```python
from build123d import *

# Parameters (mm, degrees)
SKETCH1_W             = 23.495
SKETCH1_H             = 30.48
BOSS_EXTRUDE1_DEPTH   = 3.3274
SKETCH2_W             = 21.971
SKETCH2_H             = 28.956
BOSS_EXTRUDE2_DEPTH   = 17.78
SKETCH3_W             = 16.2306
SKETCH3_H             = 24.3332
CUT_EXTRUDE1_DEPTH    = 16.51
CHAMFER1_SIZE         = 4.445
SKETCH4_W             = 4.064
SKETCH4_H             = 2.032
BOSS_EXTRUDE3_DEPTH   = 16.002
CHAMFER2_SIZE         = 1.27
CHAMFER2_SIZE2        = 0.508
CHAMFER2_PART_2_SIZE  = 1.27
CHAMFER2_PART_2_SIZE2 = 0.508
CHAMFER3_SIZE         = 1.27
CHAMFER3_SIZE2        = 0.508
CHAMFER3_PART_2_SIZE  = 1.27
CHAMFER3_PART_2_SIZE2 = 0.508
SKETCH5_W             = 4.064
SKETCH5_H             = 2.032
BOSS_EXTRUDE4_DEPTH   = 12.446
CHAMFER4_SIZE         = 1.27
CHAMFER4_SIZE2        = 0.508
CHAMFER4_PART_2_SIZE  = 1.27
CHAMFER4_PART_2_SIZE2 = 0.508
CHAMFER4_PART_3_SIZE  = 1.27
CHAMFER4_PART_3_SIZE2 = 0.508
CHAMFER4_PART_4_SIZE  = 1.27
CHAMFER4_PART_4_SIZE2 = 0.508
CHAMFER5_SIZE         = 0.508
CHAMFER5_SIZE2        = 1.27


with BuildPart() as part:
    # Sketch1 → Boss-Extrude1 (new body)
    with BuildSketch(Plane(origin=(0, 0, 0), x_dir=(0, 0, -1), z_dir=(1, 0, 0))):
        Rectangle(SKETCH1_W, SKETCH1_H)
    extrude(amount=BOSS_EXTRUDE1_DEPTH)

    # Sketch2 → Boss-Extrude2 (add)
    with BuildSketch(Plane.ZY):
        Rectangle(SKETCH2_W, SKETCH2_H)
    extrude(amount=BOSS_EXTRUDE2_DEPTH)

    # Sketch3 → Cut-Extrude1 (cut)
    with BuildSketch(Plane(origin=(3.3274, 0, 0), x_dir=(0, 0, -1), z_dir=(1, 0, 0))):
        Rectangle(SKETCH3_W, SKETCH3_H)
    extrude(amount=-CUT_EXTRUDE1_DEPTH, mode=Mode.SUBTRACT)

    # Chamfer1
    chamfer1_edges = [part.edges().sort_by_distance(p)[0] for p in [
        (-4.9276, -12.1666, 8.1153),
        (-4.9276, 12.1666, 8.1153),
    ]]
    chamfer(chamfer1_edges, length=CHAMFER1_SIZE)

    # Sketch4 → Boss-Extrude3 (add)
    with BuildSketch(Plane(origin=(2.8194, 0, 0), x_dir=(0, 0, -1), z_dir=(1, 0, 0))):
        with Locations((-4.155513801, 0.215773581)):
            Rectangle(SKETCH4_W, SKETCH4_H)
    extrude(amount=-BOSS_EXTRUDE3_DEPTH)

    # Chamfer2
    chamfer2_edges = [part.edges().sort_by_distance(p)[0] for p in [
        (2.8194, 1.231773581, 4.155513801),
    ]]
    chamfer2_side = [part.faces().sort_by_distance(p)[0] for p in [
        (-5.1816, 1.231773581, 4.155513801),
    ]]
    chamfer(chamfer2_edges, length=CHAMFER2_SIZE, length2=CHAMFER2_SIZE2, reference=chamfer2_side[0])

    # Chamfer2 part 2
    chamfer2_part_2_edges = [part.edges().sort_by_distance(p)[0] for p in [
        (2.8194, -0.800226419, 4.155513801),
    ]]
    chamfer2_part_2_side = [part.faces().sort_by_distance(p)[0] for p in [
        (-5.1816, -0.800226419, 4.155513801),
    ]]
    chamfer(chamfer2_part_2_edges, length=CHAMFER2_PART_2_SIZE, length2=CHAMFER2_PART_2_SIZE2, reference=chamfer2_part_2_side[0])

    # Chamfer3
    chamfer3_edges = [part.edges().sort_by_distance(p)[0] for p in [
        (2.8194, 0.215773581, 2.123513801),
    ]]
    chamfer3_side = [part.faces().sort_by_distance(p)[0] for p in [
        (-5.334994062, 0.215773581, 2.123513801),
    ]]
    chamfer(chamfer3_edges, length=CHAMFER3_SIZE, length2=CHAMFER3_SIZE2, reference=chamfer3_side[0])

    # Chamfer3 part 2
    chamfer3_part_2_edges = [part.edges().sort_by_distance(p)[0] for p in [
        (2.8194, 0.215773581, 6.187513801),
    ]]
    chamfer3_part_2_side = [part.faces().sort_by_distance(p)[0] for p in [
        (-5.334994062, 0.215773581, 6.187513801),
    ]]
    chamfer(chamfer3_part_2_edges, length=CHAMFER3_PART_2_SIZE, length2=CHAMFER3_PART_2_SIZE2, reference=chamfer3_part_2_side[0])

    # Sketch5 → Boss-Extrude4 (add)
    with BuildSketch(Plane(origin=(-0.7366, 0, 0), x_dir=(0, 0, -1), z_dir=(1, 0, 0))):
        with Locations((1.9685, 7.0358)):
            Rectangle(SKETCH5_W, SKETCH5_H)
    boss_extrude4 = extrude(amount=-BOSS_EXTRUDE4_DEPTH)

    # Chamfer4
    chamfer4_edges = [part.edges().sort_by_distance(p)[0] for p in [
        (-0.7366, 7.0358, -4.0005),
    ]]
    chamfer4_side = [part.faces().sort_by_distance(p)[0] for p in [
        (-6.9596, 7.0358, -4.0005),
    ]]
    chamfer(chamfer4_edges, length=CHAMFER4_SIZE, length2=CHAMFER4_SIZE2, reference=chamfer4_side[0])

    # Chamfer4 part 2
    chamfer4_part_2_edges = [part.edges().sort_by_distance(p)[0] for p in [
        (-0.7366, 8.0518, -1.9685),
    ]]
    chamfer4_part_2_side = [part.faces().sort_by_distance(p)[0] for p in [
        (-6.9596, 8.0518, -1.9685),
    ]]
    chamfer(chamfer4_part_2_edges, length=CHAMFER4_PART_2_SIZE, length2=CHAMFER4_PART_2_SIZE2, reference=chamfer4_part_2_side[0])

    # Chamfer4 part 3
    chamfer4_part_3_edges = [part.edges().sort_by_distance(p)[0] for p in [
        (-0.7366, 7.0358, 0.0635),
    ]]
    chamfer4_part_3_side = [part.faces().sort_by_distance(p)[0] for p in [
        (-6.9596, 7.0358, 0.0635),
    ]]
    chamfer(chamfer4_part_3_edges, length=CHAMFER4_PART_3_SIZE, length2=CHAMFER4_PART_3_SIZE2, reference=chamfer4_part_3_side[0])

    # Chamfer4 part 4
    chamfer4_part_4_edges = [part.edges().sort_by_distance(p)[0] for p in [
        (-0.7366, 6.0198, -1.9685),
    ]]
    chamfer4_part_4_side = [part.faces().sort_by_distance(p)[0] for p in [
        (-6.9596, 6.0198, -1.9685),
    ]]
    chamfer(chamfer4_part_4_edges, length=CHAMFER4_PART_4_SIZE, length2=CHAMFER4_PART_4_SIZE2, reference=chamfer4_part_4_side[0])

    # Mirror7: Boss-Extrude4 across plane
    add(boss_extrude4.mirror(Plane.ZX))

    # Chamfer5
    chamfer5_edges = [part.edges().sort_by_distance(p)[0] for p in [
        (-0.7366, -7.0358, -4.0005),
        (-0.7366, -8.0518, -1.9685),
        (-0.7366, -7.0358, 0.0635),
        (-0.7366, -6.0198, -1.9685),
    ]]
    chamfer5_side = [part.faces().sort_by_distance(p)[0] for p in [
        (-0.7366, -7.0358, -1.9685),
    ]]
    chamfer(chamfer5_edges, length=CHAMFER5_SIZE, length2=CHAMFER5_SIZE2, reference=chamfer5_side[0])


solid = part.part
```
For this review, take the finished solid that the model builds, in its own axes (mm). A direction names the side the tool comes from. Round coordinates to 2 decimals unless told otherwise and drop trailing zeros. Write each loop counter-clockwise with the first axis right and the second up, starting at its lowest first coordinate (ties: lowest second). Pieces come first, ordered by that corner, then holes. Notation, with made-up numbers: M 9.5,-33.5 L 25.5,-33.5 A27 cw 25.5,-6.5 Z; hole C 49,76.5 d9. An arc over 180 degrees is marked long. One line per item, written item: value. Start each with the question number.
(1) Wall thickness on line 1 (Y direction, x = -9, z = 0); line 2 (Y direction, x = -2.25, z = 3.25); line 3 (Z direction, x = -1.75, y = 3): over which ranges is each line inside the solid? List them lowest first.
(2) We need section B-B (y = 13). Give the boundary of the cut face in (x, z).
(3) The part is to be moulded in two halves that separate along Z. For faces 1 (the flat face through (-8, 6.02, -2)), 2 (the flat face through (3.327, 0, 11)), 3 (the flat face through (-9, 0, -10.986)), say which applies: released by +Z, released by -Z, zero draft, split by the parting line, or undercut.
(4) We need section A-A (x = -7.25). Give the boundary of the cut face in (y, z), and give its area (3 significant figures).
(5) Machinability: for faces 4 (the flat face through (-1.5, 7, -3.8)), 5 (the flat face through (-9, -14.478, 0)), 6 (the flat face through (2, 0, 11.748)), 7 (the flat face through (-9, 0, 10.986)), which of the approach directions +Z, -Z, +X, -X, +Y, -Y give a long, thin tool a straight path to every point of the face, cutting with its end or side? Answer none if there is none.
(6) We need section C-C (z = 8.75). Give the boundary of the cut face in (x, y), and give its area (3 significant figures).
(7) Insertion check: pin 1 (1 mm diameter, centred on x = -9.5, y = 6.5, fed in from -Z); pin 2 (4.5 mm diameter, centred on x = -7, z = -2.5, fed in from +Y); pin 3 (0.5 mm diameter, centred on y = -7, z = -1, fed in from +X). Each pin has a flat end and moves straight along its axis. Give the tip position at first contact, or say it passes through.
(8) We need section D-D (z = -2). Give the boundary of the cut face in (x, y).
Result:
1. line 1: -14.48 to -12.17, -8.05 to -6.02, 6.02 to 8.05, 12.17 to 14.48
1. line 2: -14.48 to -12.17, -0.8 to 1.23, 12.17 to 14.48
1. line 3: -10.99 to -8.12, 8.12 to 10.99
2. outline: M -17.78,-10.99 L 0,-10.99 L 0,-11.75 L 3.33,-11.75 L 3.33,11.75 L 0,11.75 L 0,10.99 L -17.78,10.99 Z
3. face 1: undercut
3. face 2: zero draft
3. face 3: released by -Z
4. outline: M -14.48,-10.99 L 14.48,-10.99 L 14.48,10.99 L -14.48,10.99 Z; M -8.05,-4 L -6.02,-4 L -6.02,0.06 L -8.05,0.06 Z; M -0.8,2.12 L 1.23,2.12 L 1.23,6.19 L -0.8,6.19 Z; M 6.02,-4 L 8.05,-4 L 8.05,0.06 L 6.02,0.06 Z; hole M -12.17,-8.12 L 12.17,-8.12 L 12.17,3.67 L 7.72,8.12 L -7.72,8.12 L -12.17,3.67 Z
4. area: 286 mm²
5. face 4: +X
5. face 5: +Z, -Z, -X, -Y
5. face 6: +Z, +X, -X, +Y, -Y
5. face 7: +Z, -X, +Y, -Y
6. outline: M -17.78,-14.48 L 0,-14.48 L 0,-15.24 L 3.33,-15.24 L 3.33,15.24 L 0,15.24 L 0,14.48 L -17.78,14.48 Z
6. area: 616 mm²
7. pin 1: z = -10.99
7. pin 2: y = 14.48
7. pin 3: x = -0.74
8. outline: M -17.78,-14.48 L 0,-14.48 L 0,-15.24 L 3.33,-15.24 L 3.33,-12.17 L -13.18,-12.17 L -13.18,-8.05 L -2.01,-8.05 L -0.74,-7.54 L -0.74,-6.53 L -2.01,-6.02 L -13.18,-6.02 L -13.18,6.02 L -2.01,6.02 L -0.74,6.53 L -0.74,7.54 L -2.01,8.05 L -13.18,8.05 L -13.18,12.17 L 3.33,12.17 L 3.33,15.24 L 0,15.24 L 0,14.48 L -17.78,14.48 Z
